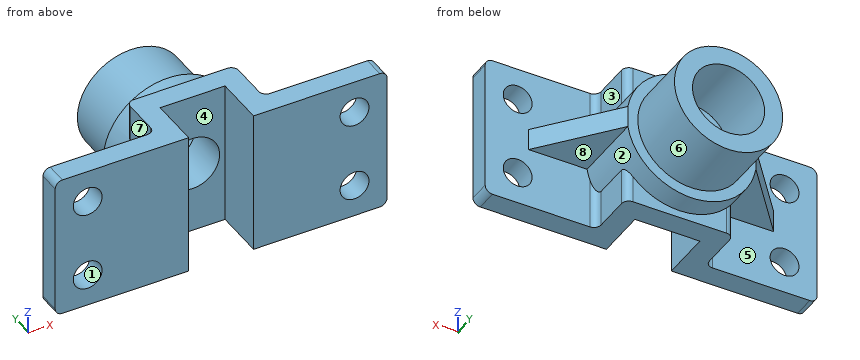
```python
from build123d import *

# Parameters (mm, degrees)
Y_KSEKLIK_EKSTR_ZYON1_DEPTH = 40
RADYUS1_R                   = 2
RADYUS2_R                   = 2
RADYUS4_R                   = 2
RADYUS5_R                   = 2
IZIM5_R                     = 4
KES_EKSTR_ZYON1_DEPTH       = 65.653926759
Y_KSEKLIK_EKSTR_ZYON3_REACH = 70.265
IZIM7_R                     = 18
IZIM8_R                     = 15
IZIM8_R_2                   = 10
Y_KSEKLIK_EKSTR_ZYON4_DEPTH = 18
IZIM9_R                     = 7.5
KES_EKSTR_ZYON3_DEPTH       = 69.265146695
IZIM12_W                    = 6
IZIM12_H                    = 20
Y_KSEKLIK_EKSTR_ZYON5_DEPTH = 19
IZIM13_W                    = 6
IZIM13_H                    = 20
Y_KSEKLIK_EKSTR_ZYON6_DEPTH = 19
KES_EKSTR_ZYON4_DEPTH       = 89.876489715


with BuildPart() as part:
    # Çizim1 → Yükseklik-Ekstrüzyon1 (new body)
    with BuildSketch(Plane.XY):
        Polygon((-43.172443791, 26.610906907), (-6.172443791, 26.610906907), (-6.172443791, 40.610906907), (11.827556209, 40.610906907), (11.827556209, 26.610906907), (48.827556209, 26.610906907), (48.827556209, 32.610906907), (17.827556209, 32.610906907), (17.827556209, 46.610906907), (-12.172443791, 46.610906907), (-12.172443791, 32.610906907), (-43.172443791, 32.610906907), align=None)
    extrude(amount=Y_KSEKLIK_EKSTR_ZYON1_DEPTH)

    # Radyus1
    radyus1_edges = [part.edges().sort_by_distance(p)[0] for p in [
        (-12.172443791, 46.610906907, 20),
        (17.827556209, 46.610906907, 20),
    ]]
    fillet(radyus1_edges, radius=RADYUS1_R)

    # Radyus2
    radyus2_edges = [part.edges().sort_by_distance(p)[0] for p in [
        (-12.172443791, 32.610906907, 20),
        (17.827556209, 32.610906907, 20),
    ]]
    fillet(radyus2_edges, radius=RADYUS2_R)

    # Radyus4
    radyus4_edges = [part.edges().sort_by_distance(p)[0] for p in [
        (-43.172443791, 29.610906907, 0),
        (48.827556209, 29.610906907, 40),
        (-43.172443791, 29.610906907, 40),
    ]]
    fillet(radyus4_edges, radius=RADYUS4_R)

    # Radyus5
    radyus5_edges = [part.edges().sort_by_distance(p)[0] for p in [
        (48.827556209, 29.610906907, 0),
    ]]
    fillet(radyus5_edges, radius=RADYUS5_R)

    # Çizim5 → Kes-Ekstrüzyon1 (cut, through all)
    with BuildSketch(Plane(origin=(0, 32.610906907, 0), x_dir=(1, 0, 0), z_dir=(0, 1, 0))):
        with Locations(Location((-34.172443791, -9, 0), (0, 0, 180))):
            Circle(IZIM5_R)
        with Locations(Location((-34.172443791, -31, 0), (0, 0, 180))):
            Circle(IZIM5_R)
        with Locations(Location((39.827556209, -9, 0), (0, 0, 180))):
            Circle(IZIM5_R)
        with Locations(Location((39.827556209, -31, 0), (0, 0, 180))):
            Circle(IZIM5_R)
    extrude(amount=-KES_EKSTR_ZYON1_DEPTH, mode=Mode.SUBTRACT)

    # Çizim7 → Yükseklik-Ekstrüzyon3 (add, up to next)
    with BuildSketch(Plane(origin=(0, 52.610906907, 0), x_dir=(1, 0, 0), z_dir=(0, 1, 0)), mode=Mode.PRIVATE) as y_kseklik_ekstr_zyon3_sk1:
        with Locations(Location((2.827556209, -20, 0), (0, 0, 180))):
            Circle(IZIM7_R)
    y_kseklik_ekstr_zyon3_tool1 = extrude(y_kseklik_ekstr_zyon3_sk1.sketch, amount=-Y_KSEKLIK_EKSTR_ZYON3_REACH, mode=Mode.PRIVATE) - part.part
    add(y_kseklik_ekstr_zyon3_tool1.solids().sort_by_distance((2.827556, 52.610907, 20))[0])

    # Çizim8 → Yükseklik-Ekstrüzyon4 (add)
    with BuildSketch(Plane(origin=(0, 52.610906907, 0), x_dir=(1, 0, 0), z_dir=(0, 1, 0))):
        with Locations(Location((2.827556209, -20, 0), (0, 0, 180))):
            Circle(IZIM8_R)
        with Locations(Location((2.827556209, -20, 0), (0, 0, 180))):
            Circle(IZIM8_R_2, mode=Mode.SUBTRACT)
    extrude(amount=Y_KSEKLIK_EKSTR_ZYON4_DEPTH)

    # Çizim9 → Kes-Ekstrüzyon3 (cut, through all)
    with BuildSketch(Plane(origin=(0, 52.610906907, 0), x_dir=(1, 0, 0), z_dir=(0, 1, 0))):
        with Locations(Location((2.827556209, -20, 0), (0, 0, 180))):
            Circle(IZIM9_R)
    extrude(amount=-KES_EKSTR_ZYON3_DEPTH, mode=Mode.SUBTRACT)

    # Çizim12 → Yükseklik-Ekstrüzyon5 (add)
    with BuildSketch(Plane.ZY.offset(12.172443791)):
        with Locations((20, 42.610906907)):
            Rectangle(IZIM12_W, IZIM12_H)
    extrude(amount=Y_KSEKLIK_EKSTR_ZYON5_DEPTH)

    # Çizim13 → Yükseklik-Ekstrüzyon6 (add)
    with BuildSketch(Plane(origin=(17.827556209, 0, 0), x_dir=(0, 0, -1), z_dir=(1, 0, 0))):
        with Locations((-20, 42.610906907)):
            Rectangle(IZIM13_W, IZIM13_H)
    extrude(amount=Y_KSEKLIK_EKSTR_ZYON6_DEPTH)

    # Çizim14 → Kes-Ekstrüzyon4 (cut, through all)
    with BuildSketch(Plane.XY.offset(23)):
        Polygon((-14.920683141, 52.610906907), (-31.172443791, 32.610906907), (-51.091158716, 48.796616278), (-34.839398065, 68.796616278), align=None)
        Polygon((20.575795558, 52.610906907), (36.827556209, 32.610906907), (59.044395874, 50.664044939), (42.792635223, 70.664044939), align=None)
    extrude(amount=-KES_EKSTR_ZYON4_DEPTH, mode=Mode.SUBTRACT)


solid = part.part
```
Source: CAD feature listing. Evaluate the final solid. Frame: model axes, mm. Face numbers are marked on the shaded views. A direction names the side the tool comes from. Coordinates: 2 decimals unless noted, no trailing zeros. Write each loop counter-clockwise with the first axis right and the second up, starting at its lowest first coordinate (ties: lowest second). Pieces come first, ordered by that corner, then holes. Notation, with made-up numbers: M 73,2 L 111,2 A9 cw 111,16 Z; hole C -19.75,50.5 d1. An arc over 180 degrees is marked long. Answer as a JSON object with one key per item and string values.
1. Cut plane A-A on z = 20. Output: boundary loops of the cut face in (x, y), plus the area to 3 significant figures.
Evaluation:
{"outline": "M -43.17,26.61 L -6.17,26.61 L -6.17,40.61 L -4.67,40.61 L -4.67,52.61 L -7.17,52.61 L -7.17,70.61 L -12.17,70.61 L -12.17,52.61 L -14.92,52.61 L -31.17,32.61 L -43.17,32.61 Z; M 10.33,40.61 L 11.83,40.61 L 11.83,26.61 L 48.83,26.61 L 48.83,32.61 L 36.83,32.61 L 20.58,52.61 L 17.83,52.61 L 17.83,70.61 L 12.83,70.61 L 12.83,52.61 L 10.33,52.61 Z", "area": "1,330 mm^2"}
2. Cut plane B-B on y = 37. Output: boundary loops of the cut face in (x, z).
Evaluation:
{"outline": "M -27.61,17 L -14.92,17 A18 ccw -12.17,10.05 L -12.17,0 L -6.17,0 L -6.17,40 L -12.17,40 L -12.17,29.95 A18 ccw -14.92,23 L -27.61,23 Z; M 11.83,0 L 17.83,0 L 17.83,10.05 A18 ccw 20.58,17 L 33.26,17 L 33.26,23 L 20.58,23 A18 ccw 17.83,29.95 L 17.83,40 L 11.83,40 Z"}
3. Ray query, L1, parallel to X at y = 27.95, z = 9; L2, parallel to X at y = 65, z = 20.5; L3, parallel to Z at x = 24, y = 47. Return the intervals inside material, ascending.
Evaluation:
{"L1": "-43.17 to -38.17, -30.17 to -6.17, 11.83 to 35.83, 43.83 to 48.83", "L2": "-12.16 to -7.16, 12.82 to 17.82", "L3": "17 to 23"}
4. Cut plane D-D on x = 41. Output: boundary loops of the cut face in (y, z), plus the area to 3 significant figures.
Evaluation:
{"outline": "M 26.61,0 L 32.61,0 L 32.61,5.18 L 26.61,5.18 Z; M 26.61,12.82 L 32.61,12.82 L 32.61,27.18 L 26.61,27.18 Z; M 26.61,34.82 L 32.61,34.82 L 32.61,40 L 26.61,40 Z", "area": "148 mm^2"}
5. Cut plane C-C on z = 31. State how many separate pieces and enclosed holes the cut face has, plus the area to 3 significant figures.
Evaluation:
{"separate pieces": "3", "enclosed holes": "0", "area": "1,160 mm^2"}
6. Contact query for flat-ended pins moving along their axis: P1, Ø13, axis at x = 28, y = 44, coming from the -Z side; P2, Ø2.5, axis at x = 3, z = 38, coming from the +Y side; P3, Ø11, axis at y = 40, z = 6, coming from the +X side. Output: stop coordinate, or through.
Evaluation:
{"P1": "z = 17", "P2": "y = 52.61", "P3": "x = 18.69"}
7. Access query for the marked faces 4, 5, 6, 7 and 8. Directions: +Z, -Z, +X, -X, +Y, -Y. A direction counts if a zero-diameter tool reaches every point of the face in a straight line with its end or side. Return the directions, or none.
Evaluation:
{"face 4": "+Z, -Z, -Y", "face 5": "-X, +Y", "face 6": "+Y", "face 7": "+Z, -X, +Y", "face 8": "-Z, +X, +Y"}
8. Draft query along Z for the marked faces 1, 2 and 3. Return one class per face: released by +Z, released by -Z, zero draft, split by the parting line, or undercut.
Evaluation:
{"face 1": "undercut", "face 2": "released by -Z", "face 3": "zero draft"}
